Input: part model. Units: mm. Frame: model coordinates. Round coordinates to 2 decimals unless told otherwise and drop trailing zeros. Order: outer loops, then holes, each group sorted by start corner. A loop starts at its lowest first (then second) coordinate and runs counter-clockwise, first axis right, second up. Notation, with made-up numbers: (21.25, 74) -> (50.25, 74) arc R28 ccw to (50.25, 112) -> close; hole circle Ø5 at (84, -8). An arc over 180 degrees is marked (long way). Use a Markdown table: item, result.
from build123d import *

# Parameters (mm, degrees)
SKETCH_1_W          = 130
SKETCH_1_H          = 28
EXTRUDE_1_DEPTH     = 3
CUT_EXTRUDE_1_REACH = 68.558
SKETCH_2_R          = 4.25
SKETCH_2_R_2        = 2.25
FILLET_1_RADIUS     = 14
FILLET_1_LENGTH     = 3
CUT_EXTRUDE_3_REACH = 68.558
SKETCH_4_R          = 140
FILLET_2_RADIUS     = 14
FILLET_2_LENGTH     = 3


with BuildPart() as part:
    # 草图1 → 凸台-拉伸1 (new body)
    with BuildSketch(Plane(origin=(0, 0, 0), x_dir=(1, 0, 0), z_dir=(0, 1, 0))):
        Rectangle(SKETCH_1_W, SKETCH_1_H)
    extrude(amount=EXTRUDE_1_DEPTH)

    # 草图2 → 切除-拉伸1 (cut, up to next)
    with BuildSketch(Plane(origin=(0, 3, 0), x_dir=(1, 0, 0), z_dir=(0, 1, 0)), mode=Mode.PRIVATE) as cut_extrude_1_sk1:
        with Locations(Location((-50, 0, 0), (0, 0, 270))):
            Circle(SKETCH_2_R)
    cut_extrude_1_tool1 = extrude(cut_extrude_1_sk1.sketch, amount=-CUT_EXTRUDE_1_REACH, mode=Mode.PRIVATE) & part.part
    # 草图2 → 切除-拉伸1 (cut, up to next)
    with BuildSketch(Plane(origin=(0, 3, 0), x_dir=(1, 0, 0), z_dir=(0, 1, 0)), mode=Mode.PRIVATE) as cut_extrude_1_sk2:
        with Locations(Location((50, 0, 0), (0, 0, 270))):
            Circle(SKETCH_2_R)
    cut_extrude_1_tool2 = extrude(cut_extrude_1_sk2.sketch, amount=-CUT_EXTRUDE_1_REACH, mode=Mode.PRIVATE) & part.part
    # 草图2 → 切除-拉伸1 (cut, up to next)
    with BuildSketch(Plane(origin=(0, 3, 0), x_dir=(1, 0, 0), z_dir=(0, 1, 0)), mode=Mode.PRIVATE) as cut_extrude_1_sk3:
        with Locations(Location((0, 0, 0), (0, 0, 270))):
            Circle(SKETCH_2_R_2)
    cut_extrude_1_tool3 = extrude(cut_extrude_1_sk3.sketch, amount=-CUT_EXTRUDE_1_REACH, mode=Mode.PRIVATE) & part.part
    add(cut_extrude_1_tool1.solids().sort_by_distance((-50, 3, 0))[0], mode=Mode.SUBTRACT)
    add(cut_extrude_1_tool2.solids().sort_by_distance((50, 3, 0))[0], mode=Mode.SUBTRACT)
    add(cut_extrude_1_tool3.solids().sort_by_distance((0, 3, 0))[0], mode=Mode.SUBTRACT)

    # 圆角1: full round fillet: the end face becomes a half cylinder, R = half its width
    fillet_1_face = Plane((-65, 1.5, 0), x_dir=(0, 1, 0), z_dir=(-1, 0, 0))  # on the end face: x along it, z out of the body
    fillet_1_slab = fillet_1_face.offset(-FILLET_1_RADIUS / 2) * Box(FILLET_1_LENGTH, 2 * FILLET_1_RADIUS, FILLET_1_RADIUS, mode=Mode.PRIVATE)  # the body's end, R deep
    fillet_1_round = Plane((-51, 1.5, 0), x_dir=(-1, 0, 0), z_dir=(0, 1, 0)) * Cylinder(FILLET_1_RADIUS, FILLET_1_LENGTH, mode=Mode.PRIVATE)  # its axis R under the face
    add(fillet_1_slab - fillet_1_round, mode=Mode.SUBTRACT)

    # 草图4 → 切除-拉伸3 (cut, up to next)
    with BuildSketch(Plane(origin=(0, 3, 0), x_dir=(1, 0, 0), z_dir=(0, 1, 0)), mode=Mode.PRIVATE) as cut_extrude_3_sk1:
        with Locations((0, 150)):
            Circle(SKETCH_4_R)
    cut_extrude_3_tool1 = extrude(cut_extrude_3_sk1.sketch, amount=-CUT_EXTRUDE_3_REACH, mode=Mode.PRIVATE) & part.part
    cut_extrude_3 = cut_extrude_3_tool1.solids().sort_by_distance((0, 3, -150))[0]
    add(cut_extrude_3, mode=Mode.SUBTRACT)

    # 镜向1: 切除-拉伸3 across plane
    add(cut_extrude_3.mirror(Plane.XY), mode=Mode.SUBTRACT)

    # 圆角2: full round fillet: the end face becomes a half cylinder, R = half its width
    fillet_2_face = Plane((65, 1.5, 0), x_dir=(0, -1, 0), z_dir=(1, 0, 0))  # on the end face: x along it, z out of the body
    fillet_2_slab = fillet_2_face.offset(-FILLET_2_RADIUS / 2) * Box(FILLET_2_LENGTH, 2 * FILLET_2_RADIUS, FILLET_2_RADIUS, mode=Mode.PRIVATE)  # the body's end, R deep
    fillet_2_round = Plane((51, 1.5, 0), x_dir=(1, 0, 0), z_dir=(0, -1, 0)) * Cylinder(FILLET_2_RADIUS, FILLET_2_LENGTH, mode=Mode.PRIVATE)  # its axis R under the face
    add(fillet_2_slab - fillet_2_round, mode=Mode.SUBTRACT)


solid = part.part
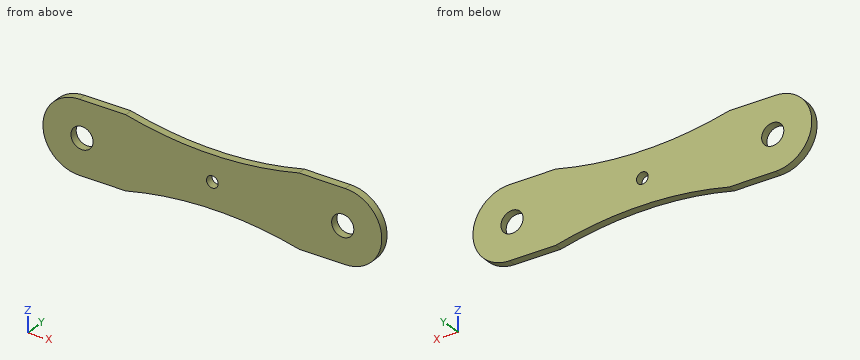
1) Cut plane D-D on z = -11.25. Return loops of the section in (x, y), and give its area (3 significant figures).
Results found:
| item | result |
|---|---|
| outline | (-59.33, 0) -> (-18.67, 0) -> (-18.67, 3) -> (-59.33, 3) -> close; (18.67, 0) -> (59.33, 0) -> (59.33, 3) -> (18.67, 3) -> close |
| area | 244 mm² |
2) Pin query (flat end, axial travel): pin 1 Ø1 at (y, z) = (2.5, -6) entering from -X; pin 2 Ø3.5 at (x, z) = (0, 0) entering from +Y. Return the tip coordinate at first contact, or that it passes through.
Results found:
| item | result |
|---|---|
| pin 1 | stops at x = -63.87 |
| pin 2 | passes through |
3) Cut plane C-C on y = 1. Return loops of the section in (x, z), and give its area (3 significant figures).
Results found:
| item | result |
|---|---|
| outline | (-51, -14) -> (-33.23, -14) arc R140 cw to (33.23, -14) -> (51, -14) arc R14 ccw to (51, 14) -> (33.23, 14) arc R140 cw to (-33.23, 14) -> (-51, 14) arc R14 ccw to start; hole circle Ø8.5 at (-50, 0); hole circle Ø4.5 at (0, 0); hole circle Ø8.5 at (50, 0) |
| area | 2,990 mm² |
4) Cut plane A-A on z = 0. Return loops of the section in (x, y), and give its area (4 significant figures).
Results found:
| item | result |
|---|---|
| outline | (-65, 0) -> (-54.25, 0) -> (-54.25, 3) -> (-65, 3) -> close; (-45.75, 0) -> (-2.25, 0) -> (-2.25, 3) -> (-45.75, 3) -> close; (2.25, 0) -> (45.75, 0) -> (45.75, 3) -> (2.25, 3) -> close; (54.25, 0) -> (65, 0) -> (65, 3) -> (54.25, 3) -> close |
| area | 325.5 mm² |
5) Line query: L1, parallel to X at y = 2.45, z = 0; L2, parallel to X at y = 1.85, z = -0.75; L3, parallel to Z at x = 17, y = 0.65. Output: solid intervals per line, ascending. Write a range as [from, to].
Results found:
| item | result |
|---|---|
| L1 | x = [-65, -54.25], [-45.75, -2.25], [2.25, 45.75], [54.25, 65] |
| L2 | x = [-64.98, -54.18], [-45.82, -2.12], [2.12, 45.82], [54.18, 64.98] |
| L3 | z = [-11.04, 11.04] |
6) Cut plane B-B on x = 0. Return loops of the section in (y, z), and give its area (3 significant figures).
Results found:
| item | result |
|---|---|
| outline | (0, -10) -> (3, -10) -> (3, -2.25) -> (0, -2.25) -> close; (0, 2.25) -> (3, 2.25) -> (3, 10) -> (0, 10) -> close |
| area | 46.5 mm² |
